Model file for the job. Use its own axes, mm. A direction names the side the tool comes from. Give positions to 0.01 mm unless a question says otherwise; leave off trailing zeros. Order: outer loops, then holes, each group sorted by start corner. A loop starts at its lowest first (then second) coordinate and runs counter-clockwise, first axis right, second up. Notation, with made-up numbers: (49.25, -27.5) -> (54.25, -27.5) arc R19 ccw to (54.25, -12.5) -> close; hole circle Ø3 at (54.5, -24.75). An arc over 180 degrees is marked (long way). Use CSV: the item, a comma, the result in double quotes. Start each with the question number.
1. Cut at A-A on z = 0. List the corners of the cut face in (x, y).
2. Cut at B-B on x = 0. List the corners of the cut face in (y, z), then the cut area to 3 significant figures.
3. Cut at C-C on y = 15. List the corners of the cut face in (x, z).
4. Pull direction Z, two halves, no side cores. Call faces 1 (the cylindrical face through (-15.821, 19.227, -20.633)), 2 (the flat face through (0, 39, 0)), 3 (the flat face through (20.5, -5, 13.1)): released by +Z, released by -Z, zero draft, split by the parting line, or undercut.
5. Drop flat-ended pins along their axis: pin 1 (14.5 mm diameter, centred on x = 11, z = 1, fed in from -Y); pin 2 (8 mm diameter, centred on x = 13.5, y = 18.5, fed in from +Z); pin 3 (8 mm diameter, centred on y = 6.5, z = 15.5, fed in from +X). Give the stop position or say it passes through.
6. Wall check: line 1 (X direction, y = 24, z = -0.5); line 2 (Y direction, x = 17, z = -12.5); line 3 (Z direction, x = -4.5, y = 19). Give the ranges that are in metal, low to high. Write a range as from..to.
7. 3-axis set-ups, long thin cutter, end or side, ignore diameter. For faces 4 (the cylindrical face through (7.509, -2.465, -23.846)), 5 (the flat face through (0, 43, 0)): which of +Z, -Z, +X, -X, +Y, -Y reach the whole face in a straight line?
```python
from build123d import *

# Parameters (mm, degrees)
SKETCH1_R           = 26
BOSS_EXTRUDE1_DEPTH = 43
SKETCH2_R           = 25
BOSS_EXTRUDE2_DEPTH = 5
SKETCH3_R           = 24.145878613
CUT_EXTRUDE1_DEPTH  = 44
FILLET1_R           = 4


with BuildPart() as part:
    # Sketch1 → Boss-Extrude1 (new body)
    with BuildSketch(Plane(origin=(0, 0, 0), x_dir=(1, 0, 0), z_dir=(0, 1, 0))):
        with Locations(Location((0, 0, 0), (0, 0, 270))):
            Circle(SKETCH1_R)
    extrude(amount=BOSS_EXTRUDE1_DEPTH)

    # Sketch2 → Boss-Extrude2 (add)
    with BuildSketch(Plane.XZ):
        with Locations(Location((0, 0, 0), (0, 0, 270))):
            Circle(SKETCH2_R)
    extrude(amount=BOSS_EXTRUDE2_DEPTH)

    # Sketch3 → Cut-Extrude1 (cut)
    with BuildSketch(Plane.XZ.offset(5)):
        with Locations(Location((0, 0, 0), (0, 0, 270))):
            Circle(SKETCH3_R)
    extrude(amount=-CUT_EXTRUDE1_DEPTH, mode=Mode.SUBTRACT)

    # Fillet1
    fillet1_edges = [part.edges().sort_by_distance(p)[0] for p in [
        (0, 43, -26),
    ]]
    fillet(fillet1_edges, radius=FILLET1_R)


solid = part.part
```
Verdict:
1,outline,"(-26, 0) -> (-25, 0) -> (-25, -5) -> (-24.15, -5) -> (-24.15, 39) -> (24.15, 39) -> (24.15, -5) -> (25, -5) -> (25, 0) -> (26, 0) -> (26, 39) arc R4 ccw to (22, 43) -> (-22, 43) arc R4 ccw to (-26, 39) -> close"
2,outline,"(-5, -25) -> (0, -25) -> (0, -26) -> (39, -26) arc R4 ccw to (43, -22) -> (43, 22) arc R4 ccw to (39, 26) -> (0, 26) -> (0, 25) -> (-5, 25) -> (-5, 24.15) -> (39, 24.15) -> (39, -24.15) -> (-5, -24.15) -> close"
2,area,"354 mm^2"
3,outline,"circle Ø52 at (0, 0); hole circle Ø48.29 at (0, 0)"
4,face 1,"split by the parting line"
4,face 2,"undercut"
4,face 3,"zero draft"
5,pin 1,"y = 39"
5,pin 2,"z = 24.2"
5,pin 3,"x = 23.32"
6,line 1,"-26..-24.14, 24.14..26"
6,line 2,"39..43"
6,line 3,"-25.61..-23.72, 23.72..25.61"
7,face 4,"-Y"
7,face 5,"+Z, -Z, +X, -X, +Y"
